Could you check a few things on this model? Use its own coordinates, in mm. Round coordinates to 2 decimals unless told otherwise and drop trailing zeros. Loops run counter-clockwise (first coordinate to the right, second up) from the corner with the lowest first, then second, coordinate; pieces in that order, holes last. Notation, with made-up numbers: (50, -40) -> (87, -40) arc R19 cw to (87, -5) -> close; hole circle Ø2 at (-23, 7.5). An arc over 180 degrees is marked (long way). Put each result on its own line as item: value. Start each with the question number.
1. Imagine slicing it at A-A, the plane z = -40. Please give me the cut outline in (x, y), and give its area (3 significant figures).
2. Imagine slicing it at D-D, the plane z = 15. Please give me the cut outline in (x, y), and give its area (3 significant figures).
3. Imagine slicing it at B-B, the plane z = -5.15. Please give me the cut outline in (x, y).
4. I need wall thicknesses on line 1 (X direction, y = 2.1, z = -5.15); line 2 (Z direction, x = -19.5, y = 2); line 3 (X direction, y = 2.5, z = 15). Which ranges of each line are inside material? Lowest first, please. Write a range as [from, to].
5. Imagine slicing it at C-C, the plane x = -27. Please give me the cut outline in (y, z), and give its area (3 significant figures).
6. I'm going to push flat-ended pins straight in: P1, Ø5, axis at x = -3, z = -8, coming from the -Y side; P2, Ø2, axis at y = 1.5, z = 39.5, coming from the +X side; P3, Ø2, axis at y = 1.5, z = -48.5, coming from the -X side; P4, Ø1, axis at x = 7, y = 2, coming from the -Z side. Where does each tip first touch, or does it pass through?
Autodesk Inventor part; units mm, degrees
ref_plane "YZ Plane" through (0, 0, 0) normal (1, 0, 0) x (0, 1, 0)
ref_plane "XZ Plane" through (0, 0, 0) normal (0, 1, 0) x (-1, 0, 0)
ref_plane "XY Plane" through (0, 0, 0) normal (0, 0, 1) x (1, 0, 0)
sketch "Sketch1" plane through (0, 0, 0) normal (0, 1, 0) x (-1, 0, 0)
  line L0 (-17.5, 50) -> (17.5, 50)
  line L1 (17.5, 50) -> (17.5, -50)
  line L2 (17.5, -50) -> (-17.5, -50)
  line L3 (-17.5, -50) -> (-17.5, 50)
  line L4 (-17.5, 50) -> (17.5, -50) construction
  line L5 (17.5, 50) -> (-17.5, -50) construction
  line L6 (7.5, 50) -> (0, 50)
  line L7 (0, 50) -> (0, 54)
  line L8 (0, 54) -> (7.5, 54)
  line L9 (7.5, 54) -> (7.5, 50)
  line L10 (-10, 50) -> (-21.5, 50)
  line L11 (-21.5, 50) -> (-21.5, 54)
  line L12 (-21.5, 54) -> (-10, 54)
  line L13 (-10, 54) -> (-10, 50)
  line L14 (17.5, 30) -> (21.5, 30)
  line L15 (21.5, 30) -> (21.5, 0)
  line L16 (21.5, 0) -> (17.5, 0)
  line L17 (17.5, 0) -> (17.5, 30)
  line L18 (17.5, -20) -> (21.5, -20)
  line L19 (21.5, -20) -> (21.5, -54)
  line L20 (21.5, -54) -> (17.5, -54)
  line L21 (17.5, -54) -> (17.5, -20)
  line L22 (7.5, -50) -> (0, -50)
  line L23 (0, -50) -> (0, -54)
  line L24 (0, -54) -> (7.5, -54)
  line L25 (7.5, -54) -> (7.5, -50)
  line L26 (-10, -50) -> (-21.5, -50)
  line L27 (-21.5, -50) -> (-21.5, -54)
  line L28 (-21.5, -54) -> (-10, -54)
  line L29 (-10, -54) -> (-10, -50)
  line L30 (-17.5, 30) -> (-21.5, 30)
  line L31 (-21.5, 30) -> (-21.5, 0)
  line L32 (-21.5, 0) -> (-17.5, 0)
  line L33 (-17.5, 0) -> (-17.5, 30)
  line L34 (-17.5, -50) -> (-21.5, -50)
  line L35 (-21.5, -50) -> (-21.5, -20)
  line L36 (-21.5, -20) -> (-17.5, -20)
  line L37 (-17.5, -20) -> (-17.5, -50)
  point P0 (0, 0)
  point P1 (17.5, 0)
  point P2 (-17.5, 0)
  point P3 (-17.5, -20)
  point P4 (-21.5, -50)
  point P5 (0, -50)
  point P6 (17.5, -50)
  dimension "d0" = 35
  dimension "d2" = 7.5
  dimension "d3" = 4
  dimension "d4" = 11.5
  dimension "d5" = 4
  dimension "d6" = 10
  dimension "d7" = 10
  dimension "d8" = 4
  dimension "d9" = 30
  dimension "d10" = 4
  dimension "d11" = 34
  dimension "d12" = 20
  dimension "d13" = 20
  dimension "d14" = 7.5
  dimension "d15" = 4
  dimension "d16" = 11.5
  dimension "d17" = 4
  dimension "d18" = 10
  dimension "d19" = 10
  dimension "d20" = 4
  dimension "d21" = 30
  dimension "d22" = 20
  dimension "d23" = 4
  dimension "d24" = 30
  dimension "d27" = 4
extrude "Extrusion1" add sketch "Sketch1" along normal blind 4
sketch "Sketch2" plane through (0, 4, 0) normal (0, 1, 0) x (1, 0, 0)
  line L0 (-21.5, 54) -> (-33.5, 54)
  line L1 (-33.5, 54) -> (-33.5, -54)
  line L2 (-33.5, -54) -> (-21.5, -54)
  line L3 (-21.5, -54) -> (-21.5, 54)
  line L4 (-7.5, -54) -> (0, -54)
  line L5 (-21.5, 54) -> (-21.5, 20)
  line L6 (-21.5, 20) -> (-17.5, 20)
  line L7 (-17.5, 20) -> (-17.5, 0)
  line L8 (-17.5, 0) -> (-21.5, 0)
  line L9 (-21.5, 0) -> (-21.5, -30)
  line L10 (-21.5, -30) -> (-17.5, -30)
  line L11 (-17.5, -30) -> (-17.5, -50)
  line L12 (-17.5, -50) -> (-7.5, -50)
  line L13 (-7.5, -50) -> (-7.5, -54)
  line L14 (-7.5, -54) -> (0, -54)
  line L15 (0, -54) -> (0, -50)
  line L16 (0, -50) -> (10, -50)
  line L17 (10, -50) -> (10, -54)
  line L18 (10, -54) -> (21.5, -54)
  line L19 (21.5, -54) -> (21.5, -50)
  line L20 (21.5, -50) -> (17.5, -50)
  line L21 (17.5, -50) -> (17.5, -30)
  line L22 (17.5, -30) -> (21.5, -30)
  line L23 (21.5, -30) -> (21.5, 0)
  line L24 (21.5, 0) -> (17.5, 0)
  line L25 (17.5, 0) -> (17.5, 20)
  line L26 (17.5, 20) -> (21.5, 20)
  line L27 (21.5, 20) -> (21.5, 54)
  line L28 (21.5, 54) -> (10, 54)
  line L29 (10, 54) -> (10, 50)
  line L30 (10, 50) -> (0, 50)
  line L31 (0, 50) -> (0, 54)
  line L32 (0, 54) -> (-7.5, 54)
  line L33 (-7.5, 54) -> (-7.5, 50)
  line L34 (-7.5, 50) -> (-17.5, 50)
  line L35 (-17.5, 50) -> (-17.5, 54)
  line L36 (-17.5, 54) -> (-21.5, 54)
  line L37 (-29.5, 30) -> (-25.5, 30)
  line L38 (-25.5, 30) -> (-25.5, 10)
  line L39 (-25.5, 10) -> (-29.5, 10)
  line L40 (-29.5, 10) -> (-29.5, 30)
  line L41 (-25.5, -30) -> (-29.5, -30)
  line L42 (-29.5, -30) -> (-29.5, -10)
  line L43 (-29.5, -10) -> (-25.5, -10)
  line L44 (-25.5, -10) -> (-25.5, -30)
  line L45 (-29.5, 10) -> (-25.5, -10) construction
  point P0 (0, 0)
  point P1 (-27.5, 0)
  point P2 (-33.5, 0)
  dimension "d29" = 4
  dimension "d30" = 20
  dimension "d31" = 20
  dimension "d32" = 4
  dimension "d35" = 51
extrude "Extrusion2" add sketch "Sketch2" against normal up to surface (4 mm away) contours L3 L2 L1 L0
sketch "Sketch3" plane through (0, 4, 0) normal (0, 1, 0) x (1, 0, 0)
  line L0 (-1.8, 2) -> (-1.8, 8.3) construction
  line L1 (17.5, 0) -> (17.5, 20)
  line L2 (-21.5, -30) -> (-17.5, -30)
  line L3 (-17.5, -30) -> (-17.5, -50)
  line L4 (-17.5, -50) -> (-7.5, -50)
  line L5 (-7.5, -50) -> (-7.5, -54)
  line L6 (-7.5, -54) -> (0, -54)
  line L7 (0, -54) -> (0, -50)
  line L8 (0, -50) -> (10, -50)
  line L9 (10, -50) -> (10, -54)
  line L10 (10, -54) -> (21.5, -54)
  line L11 (21.5, -54) -> (21.5, -50)
  line L12 (21.5, -50) -> (17.5, -50)
  line L13 (17.5, -50) -> (17.5, -30)
  line L14 (17.5, -30) -> (21.5, -30)
  line L15 (21.5, -30) -> (21.5, 0)
  line L16 (21.5, 0) -> (17.5, 0)
  line L17 (17.5, 0) -> (17.5, 20)
  line L18 (17.5, 20) -> (21.5, 20)
  line L19 (21.5, 20) -> (21.5, 54)
  line L20 (21.5, 54) -> (10, 54)
  line L21 (10, 54) -> (10, 50)
  line L22 (10, 50) -> (0, 50)
  line L23 (0, 50) -> (0, 54)
  line L24 (0, 54) -> (-7.5, 54)
  line L25 (-7.5, 54) -> (-7.5, 50)
  line L26 (-7.5, 50) -> (-17.5, 50)
  line L27 (-17.5, 50) -> (-17.5, 54)
  line L28 (-17.5, 54) -> (-33.5, 54)
  line L29 (-33.5, 54) -> (-33.5, -54)
  line L30 (-33.5, -54) -> (-21.5, -54)
  line L31 (-21.5, -54) -> (-21.5, -30)
  line L32 (-25.5, -30) -> (-29.5, -30)
  line L33 (-29.5, -30) -> (-29.5, -10)
  line L34 (-29.5, -10) -> (-25.5, -10)
  line L35 (-25.5, -10) -> (-25.5, -30)
  line L36 (-29.5, 30) -> (-25.5, 30)
  line L37 (-25.5, 30) -> (-25.5, 10)
  line L38 (-25.5, 10) -> (-29.5, 10)
  line L39 (-29.5, 10) -> (-29.5, 30)
  line L40 (-21.5, 0) -> (-21.5, 20)
  line L41 (-21.5, 20) -> (-17.5, 20)
  line L42 (-17.5, 20) -> (-17.5, 0)
  line L43 (-17.5, 0) -> (-21.5, 0)
  line L44 (-25.5, 10) -> (-29.5, 10)
  line L45 (-25.5, -30) -> (-25.5, -10)
  line L46 (-29.5, 10) -> (-25.5, -10) construction
  point P0 (0, 0)
  point P1 (-27.5, 0)
  point P2 (6.15, 5.15)
  point P3 (-12.85, 5.15)
  point P4 (-1.8, 5.15)
  dimension "d36" = 19.3
  dimension "d37" = 6.3
  dimension "d38" = 2
  dimension "d39" = 7.95
  dimension "d40" = 11.05
hole "Hole1" at (-12.85, 4, -5.15) at (6.15, 4, -5.15) direction (0, -1, 0) diameter 3.1 depth 4
sketch "Sketch4" plane through (0, 4, 0) normal (0, 1, 0) x (1, 0, 0)
  circle A0 centre (-12.85, 5.15) radius 1.55
  circle A1 centre (6.15, 5.15) radius 1.55
  line L0 (-21.5, -30) -> (-17.5, -30)
  line L1 (-17.5, -30) -> (-17.5, -50)
  line L2 (-17.5, -50) -> (-7.5, -50)
  line L3 (-7.5, -50) -> (-7.5, -54)
  line L4 (-7.5, -54) -> (0, -54)
  line L5 (0, -54) -> (0, -50)
  line L6 (0, -50) -> (10, -50)
  line L7 (10, -50) -> (10, -54)
  line L8 (10, -54) -> (21.5, -54)
  line L9 (21.5, -54) -> (21.5, -50)
  line L10 (21.5, -50) -> (17.5, -50)
  line L11 (17.5, -50) -> (17.5, -30)
  line L12 (17.5, -30) -> (21.5, -30)
  line L13 (21.5, -30) -> (21.5, 0)
  line L14 (21.5, 0) -> (17.5, 0)
  line L15 (17.5, 0) -> (17.5, 20)
  line L16 (17.5, 20) -> (21.5, 20)
  line L17 (21.5, 20) -> (21.5, 54)
  line L18 (21.5, 54) -> (10, 54)
  line L19 (10, 54) -> (10, 50)
  line L20 (10, 50) -> (0, 50)
  line L21 (0, 50) -> (0, 54)
  line L22 (0, 54) -> (-7.5, 54)
  line L23 (-7.5, 54) -> (-7.5, 50)
  line L24 (-7.5, 50) -> (-17.5, 50)
  line L25 (-17.5, 50) -> (-17.5, 54)
  line L26 (-17.5, 54) -> (-33.5, 54)
  line L27 (-33.5, 54) -> (-33.5, -54)
  line L28 (-33.5, -54) -> (-21.5, -54)
  line L29 (-21.5, -54) -> (-21.5, -30)
  line L30 (-25.5, -30) -> (-29.5, -30)
  line L31 (-29.5, -30) -> (-29.5, -10)
  line L32 (-29.5, -10) -> (-25.5, -10)
  line L33 (-25.5, -10) -> (-25.5, -30)
  line L34 (-29.5, 30) -> (-25.5, 30)
  line L35 (-25.5, 30) -> (-25.5, 10)
  line L36 (-25.5, 10) -> (-29.5, 10)
  line L37 (-29.5, 10) -> (-29.5, 30)
  line L38 (-21.5, 0) -> (-21.5, 20)
  line L39 (-21.5, 20) -> (-17.5, 20)
  line L40 (-17.5, 20) -> (-17.5, 0)
  line L41 (-17.5, 0) -> (-21.5, 0)
  line L42 (-9.85, 8.65) -> (3.15, 8.65)
  line L43 (3.15, 8.65) -> (3.15, 1.65)
  line L44 (3.15, 1.65) -> (-9.85, 1.65)
  line L45 (-9.85, 1.65) -> (-9.85, 8.65)
  line L46 (-12.85, 5.15) -> (-9.85, 5.15) construction
  line L47 (3.15, 5.15) -> (6.15, 5.15) construction
  point P0 (0, 0)
  dimension "d49" = 7
  dimension "d54" = 3
extrude "Extrusion3" cut sketch "Sketch4" against normal through all contours L42 L43 L44 L45
sketch "Sketch5" plane through (0, 4, 0) normal (0, 1, 0) x (1, 0, 0)
  line L0 (12.7, 11.5) -> (17.5, 11.5)
  line L1 (17.5, 11.5) -> (17.5, 20) construction
  line L2 (17.5, 20) -> (21.5, 20) construction
  line L3 (21.5, 20) -> (21.5, 54) construction
  line L4 (21.5, 54) -> (10, 54) construction
  line L5 (10, 54) -> (10, 50) construction
  line L6 (10, 50) -> (6.5, 50) construction
  line L7 (6.5, 50) -> (6.5, 45.2)
  line L8 (6.5, 45.2) -> (7.7, 45.2)
  line L9 (7.7, 45.2) -> (7.7, 42.8)
  line L10 (7.7, 42.8) -> (6.5, 42.8)
  line L11 (6.5, 42.8) -> (6.5, 38)
  line L12 (6.5, 38) -> (3.5, 38)
  line L13 (3.5, 38) -> (3.5, 42.8)
  line L14 (3.5, 42.8) -> (2.3, 42.8)
  line L15 (2.3, 42.8) -> (2.3, 45.2)
  line L16 (2.3, 45.2) -> (3.5, 45.2)
  line L17 (3.5, 45.2) -> (3.5, 50)
  line L18 (3.5, 50) -> (0, 50) construction
  line L19 (0, 50) -> (0, 54) construction
  line L20 (0, 54) -> (-7.5, 54) construction
  line L21 (-7.5, 54) -> (-7.5, 50) construction
  line L22 (-7.5, 50) -> (-17.5, 50) construction
  line L23 (-17.5, 50) -> (-17.5, 54) construction
  line L24 (-17.5, 54) -> (-33.5, 54) construction
  line L25 (-33.5, 54) -> (-33.5, -54) construction
  line L26 (-33.5, -54) -> (-21.5, -54) construction
  line L27 (-21.5, -54) -> (-21.5, -30) construction
  line L28 (-21.5, -30) -> (-17.5, -30) construction
  line L29 (-17.5, -30) -> (-17.5, -50) construction
  line L30 (-17.5, -50) -> (-7.5, -50) construction
  line L31 (-7.5, -50) -> (-7.5, -54) construction
  line L32 (-7.5, -54) -> (0, -54) construction
  line L33 (0, -54) -> (0, -50)
  line L34 (0, -50) -> (3.5, -50)
  line L35 (3.5, -50) -> (3.5, -45.2)
  line L36 (3.5, -45.2) -> (2.3, -45.2)
  line L37 (2.3, -45.2) -> (2.3, -42.8)
  line L38 (2.3, -42.8) -> (3.5, -42.8)
  line L39 (3.5, -42.8) -> (3.5, -38)
  line L40 (3.5, -38) -> (6.5, -38)
  line L41 (6.5, -38) -> (6.5, -42.8)
  line L42 (6.5, -42.8) -> (7.7, -42.8)
  line L43 (7.7, -42.8) -> (7.7, -45.2)
  line L44 (7.7, -45.2) -> (6.5, -45.2)
  line L45 (6.5, -45.2) -> (6.5, -50)
  line L46 (6.5, -50) -> (10, -50) construction
  line L47 (10, -50) -> (10, -54) construction
  line L48 (10, -54) -> (21.5, -54) construction
  line L49 (21.5, -54) -> (21.5, -50) construction
  line L50 (21.5, -50) -> (17.5, -50) construction
  line L51 (17.5, -50) -> (17.5, -30) construction
  line L52 (17.5, -30) -> (21.5, -30) construction
  line L53 (21.5, 0) -> (17.5, 0) construction
  line L54 (17.5, 0) -> (17.5, 8.5) construction
  line L55 (17.5, 8.5) -> (12.7, 8.5)
  line L56 (12.7, 8.5) -> (12.7, 7.3)
  line L57 (12.7, 7.3) -> (10.3, 7.3)
  line L58 (10.3, 7.3) -> (10.3, 8.5)
  line L59 (10.3, 8.5) -> (5.5, 8.5)
  line L60 (5.5, 8.5) -> (5.5, 11.5)
  line L61 (5.5, 11.5) -> (10.3, 11.5)
  line L62 (10.3, 11.5) -> (10.3, 12.7)
  line L63 (10.3, 12.7) -> (12.7, 12.7)
  line L64 (12.7, 12.7) -> (12.7, 11.5)
  circle A0 centre (-19.5, -15) radius 1.5
  line L65 (-29.5, 10) -> (-25.5, 10) construction
  line L66 (-25.5, 10) -> (-25.5, -10) construction
  line L67 (-25.5, -10) -> (-29.5, -10) construction
  line L68 (-29.5, -10) -> (-29.5, 10) construction
  line L69 (-21.5, 0) -> (-21.5, 20) construction
  line L70 (-21.5, 20) -> (-17.5, 20) construction
  line L71 (-17.5, 20) -> (-17.5, 0) construction
  line L72 (-17.5, 0) -> (-21.5, 0) construction
  line L73 (3.5, 50) -> (6.5, 50)
  line L74 (10, 50) -> (0, 50)
  line L75 (17.5, 11.5) -> (17.5, 8.5)
  line L76 (3.5, -50) -> (6.5, -50)
  line L77 (0, -50) -> (10, -50)
  point P0 (0, 0)
extrude "Extrusion4" cut sketch "Sketch5" against normal up to next
fillet "Fillet1" radius 12 2 edges at (-33.5, 2, 54) (-33.5, 2, -54)
properties part number "FloorButtonHolder_Top_V1_B" material "MDF Medium Density Fiberboard"
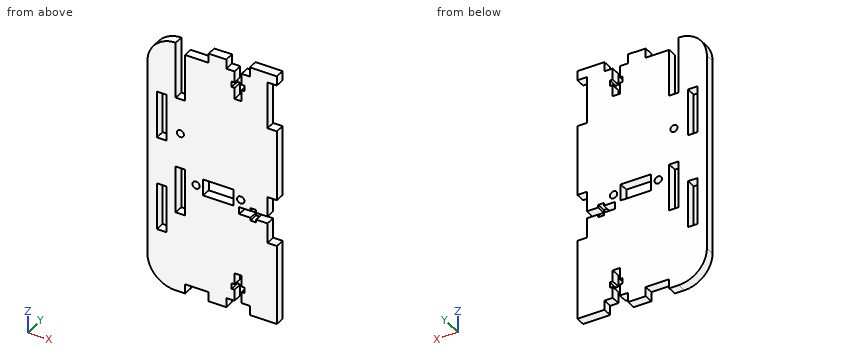
Entries:
1. outline: (-33.5, 0) -> (3.5, 0) -> (3.5, 4) -> (-33.5, 4) -> close; (6.5, 0) -> (21.5, 0) -> (21.5, 4) -> (6.5, 4) -> close
1. area: 208 mm^2
2. outline: (-33.5, 0) -> (-29.5, 0) -> (-29.5, 4) -> (-33.5, 4) -> close; (-25.5, 0) -> (-21, 0) -> (-21, 4) -> (-25.5, 4) -> close; (-18, 0) -> (21.5, 0) -> (21.5, 4) -> (-18, 4) -> close
2. area: 192 mm^2
3. outline: (-33.5, 0) -> (-21.5, 0) -> (-21.5, 4) -> (-33.5, 4) -> close; (-17.5, 0) -> (-14.4, 0) -> (-14.4, 4) -> (-17.5, 4) -> close; (-11.3, 0) -> (-9.85, 0) -> (-9.85, 4) -> (-11.3, 4) -> close; (3.15, 0) -> (4.6, 0) -> (4.6, 4) -> (3.15, 4) -> close; (7.7, 0) -> (17.5, 0) -> (17.5, 4) -> (7.7, 4) -> close
4. line 1: [-33.5, -21.5], [-17.5, -14.4], [-11.3, -9.85], [3.15, 4.6], [7.7, 17.5]
4. line 2: [-54, -20], [0, 13.5], [16.5, 30]
4. line 3: [-33.5, -29.5], [-25.5, -21], [-18, 21.5]
5. outline: (0, -52.67) -> (4, -52.67) -> (4, -30) -> (0, -30) -> close; (0, -10) -> (4, -10) -> (4, 10) -> (0, 10) -> close; (0, 30) -> (4, 30) -> (4, 52.67) -> (0, 52.67) -> close
5. area: 261 mm^2
6. P1: y = 0
6. P2: x = 17.5
6. P3: x = -32.17
6. P4: z = -50
